Verification items for the finished model (mm, model axes). Face numbers are marked on the shaded views. A direction names the side the tool comes from. Give positions to 0.01 mm unless a question says otherwise; leave off trailing zeros. Loops run counter-clockwise (first coordinate to the right, second up) from the corner with the lowest first, then second, coordinate; pieces in that order, holes last. Notation, with made-up numbers: M 79,28.5 L 102,28.5 A24 ccw 102,62.5 Z; hole C 85,25.25 d11. An arc over 180 degrees is marked long. Use a Markdown table: item, result.
from build123d import *

# Parameters (mm, degrees)
F2_R     = 0.8
F3_SIZE  = 0.8
F5_DEPTH = 2
F6_SIZE2 = 0.25
F6_SIZE  = 0.4330127019


with BuildPart() as f1:
    # F0 (on Front) → F1 (revolve)
    with BuildSketch(Plane.XZ):
        Polygon((-2.5, 0), (0, 0), (0, 17.2783121635), (-1.25, 18), (-1.25, 21), (-4.25, 21), (-4.25, 16), (-2.5, 16), (-2.5, 13.6), (-2, 13.35), (-2.5, 13.1), align=None)
    revolve(axis=Axis((0, 0, 18.332445994), (0, 0, 1)))

    # F2
    f2_edges = [f1.edges().sort_by_distance(p)[0] for p in [
        (4.25, 0, 21),
    ]]
    fillet(f2_edges, radius=F2_R)

    # F3
    f3_edges = [f1.edges().sort_by_distance(p)[0] for p in [
        (2.5, 0, 0),
    ]]
    chamfer(f3_edges, length=F3_SIZE)

    # F4 (on face) → F5 (cut)
    with BuildSketch(Plane.XY.offset(21)):
        Polygon((-1.1547005384, -2), (1.1547005384, -2), (2.3094010768, 0), (1.1547005384, 2), (-1.1547005384, 2), (-2.3094010768, 0), align=None)
    extrude(amount=-F5_DEPTH, mode=Mode.SUBTRACT)

    # F6
    f6_edges = [f1.edges().sort_by_distance(p)[0] for p in [
        (1.25, 0, 19),
    ]]
    f6_side = f1.faces().sort_by_distance((-1.679136, -0.969449, 19))[0]
    chamfer(f6_edges, length=F6_SIZE, length2=F6_SIZE2, reference=f6_side)


solid = f1.part
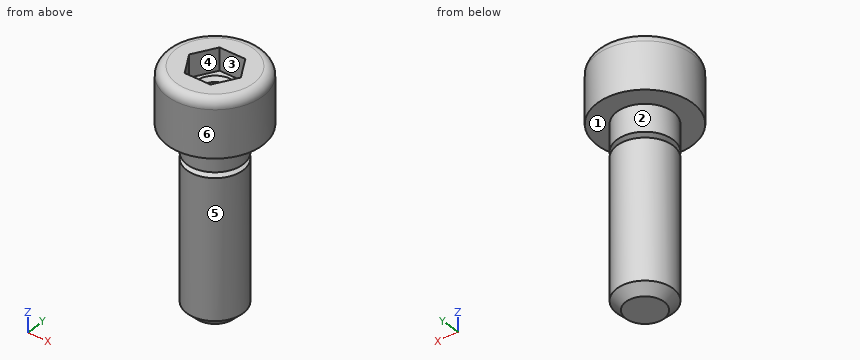
(1) Gauge pin test, flat ends, axial feed: P1, Ø3, axis at y = -1, z = 14, coming from the +X side; P2, Ø2, axis at y = 2.5, z = 16, coming from the +X side; P3, Ø1.5, axis at x = 0.5, z = 5, coming from the +Y side. Record the tip position at first contact, or that the pin passes through.
Results below:
| item | result |
|---|---|
| P1 | x = 2.5 |
| P2 | x = 3.98 |
| P3 | y = 2.5 |
(2) Material ranges on line 1 (X direction, y = 0, z = 18.45); line 2 (Z direction, x = -3, y = 0.75), recorded low to high.
Results below:
| item | result |
|---|---|
| line 1 | -4.25 to -1.25, 1.25 to 4.25 |
| line 2 | 16 to 21 |
(3) Set-up check for the marked faces 5 and 6: record each of +Z, -Z, +X, -X, +Y, -Y from which the full face is reachable in a straight line by a thin tool's end or side.
Results below:
| item | result |
|---|---|
| face 5 | -Z |
| face 6 | +Z, -Z |
(4) Draft check along Y on the marked faces 1, 2, 3 and 4. Enter one of: +Y half, -Y half, draft (parallel to the pull), parting line (faces both ways), or undercut.
Results below:
| item | result |
|---|---|
| face 1 | draft |
| face 2 | parting line |
| face 3 | undercut |
| face 4 | undercut |
(5) Cross-section at A-A on z = 17.5. Record the cut outline in (x, y).
Results below:
| item | result |
|---|---|
| outline | C 0,0 d8.5; hole C 0,0 d0.77 |
